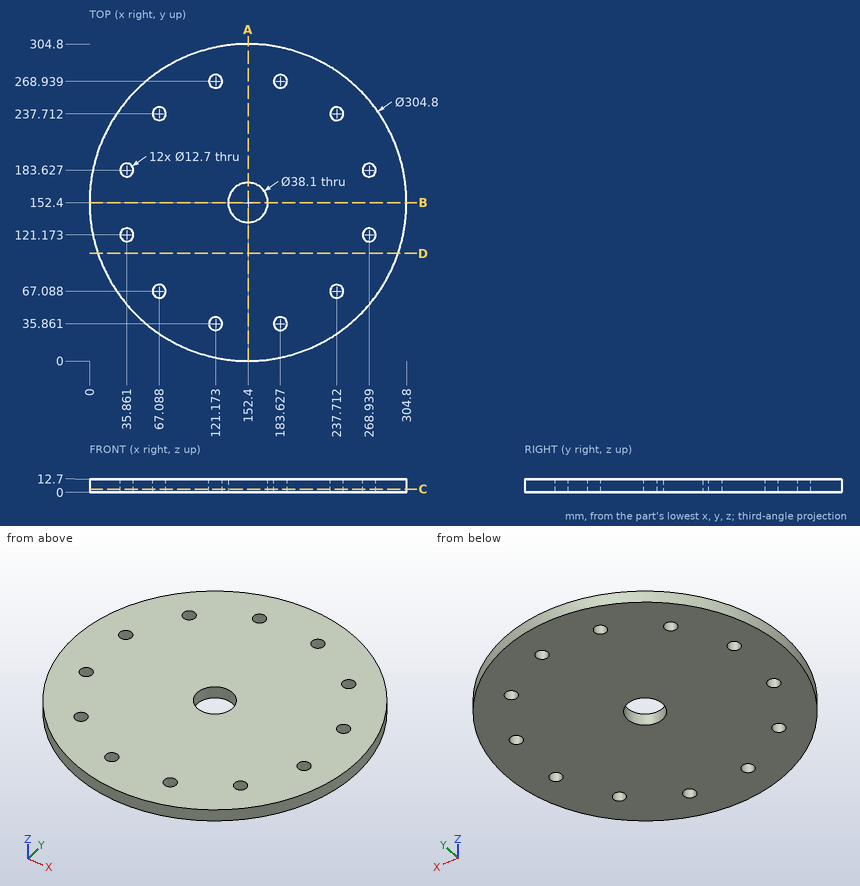
The drawing under review shows one solid part. Ordinate dimensions are in mm from its lowest x, y, z. Coordinates: 2 decimals unless noted, no trailing zeros. Write each loop counter-clockwise with the first axis right and the second up, starting at its lowest first coordinate (ties: lowest second). Pieces come first, ordered by that corner, then holes. Notation, with made-up numbers: (54, 70) -> (91, 70) arc R23 ccw to (91, 91) -> close; hole circle Ø1 at (6, 59.25). An arc over 180 degrees is marked (long way). One line per item, written item: value. Start each with the question number.
Q1. To check wall thickness, follow probe 1 along X at (y, z) = (35.5, 3) (1 decimal); probe 2 along Y at (x, z) = (235, 9.5) (1 decimal); probe 3 along Y at (x, z) = (269, 9.5) (1 decimal). State the ranges of each line that lie inside material, in increasing order.
Q2. Clearance check with flat-ended pins moving along their axes: P1, Ø2, axis at y = 81, z = 10.5, coming from the -X side (1 decimal); P2, Ø7.5, axis at x = 35.86, y = 121.17, coming from the +Z side; P3, Ø2, axis at x = 82, z = 10, coming from the -Y side; P4, Ø3, axis at y = 48.5, z = 5, coming from the -X side. State where each tip first meets the part, or that it passes through.
Q3. Add section D-D, the plane y = 103.5. Give the boundary of the cut face in (x, z), then the cut area to 3 significant figures.
Q4. Add section C-C, the plane z = 3. Count the separate pieces of the cut face and the enclosed holes in it, then the cut area to 3 significant figures.
Q5. Add section A-A, the plane x = 152.4. Give the boundary of the cut face in (y, z).
Response:
1. probe 1: 54.6 to 114.8, 127.5 to 177.3, 190 to 250.2
1. probe 2: 24.3 to 61.3, 72.8 to 232, 243.5 to 280.5
1. probe 3: 54.3 to 114.8, 127.5 to 177.3, 190 to 250.5
2. P1: x = 17.2
2. P2: through
2. P3: y = 16.72
2. P4: x = 39.53
3. outline: (8.06, 0) -> (296.74, 0) -> (296.74, 12.7) -> (8.06, 12.7) -> close
3. area: 3,670 mm²
4. separate pieces: 1
4. enclosed holes: 13
4. area: 70,300 mm²
5. outline: (0, 0) -> (133.35, 0) -> (133.35, 12.7) -> (0, 12.7) -> close; (171.45, 0) -> (304.8, 0) -> (304.8, 12.7) -> (171.45, 12.7) -> close
